Autodesk Inventor part; units mm, degrees
ref_plane "YZ Plane" through (0, 0, 0) normal (1, 0, 0) x (0, 1, 0)
ref_plane "XZ Plane" through (0, 0, 0) normal (0, 1, 0) x (-1, 0, 0)
ref_plane "XY Plane" through (0, 0, 0) normal (0, 0, 1) x (1, 0, 0)
sketch "Sketch1" plane through (0, 0, 0) normal (0, 0, 1) x (1, 0, 0)
  line L0 (55, -30) -> (-55, -30)
  line L1 (-55, -30) -> (-55, 30)
  line L2 (-55, 30) -> (55, 30)
  line L3 (55, 30) -> (55, -30)
  line L4 (49.5, -24.5) -> (-49.5, -24.5)
  line L5 (-49.5, -24.5) -> (-49.5, 24.5)
  line L6 (-49.5, 24.5) -> (49.5, 24.5)
  line L7 (49.5, 24.5) -> (49.5, -24.5)
  line L8 (55, 0) -> (-55, 0) construction
  line L9 (0, -30) -> (0, 30) construction
  line L10 (-35, 30) -> (-35, 24.5)
  line L11 (-55, 15) -> (-49.5, 15)
  line L12 (35, -24.5) -> (35, -30)
  line L13 (49.5, -15) -> (55, -15)
  line L14 (-35, -24.5) -> (-35, -30)
  line L15 (-55, -15) -> (-49.5, -15)
  line L16 (35, 30) -> (35, 24.5)
  line L17 (49.5, 15) -> (55, 15)
  line L18 (-52.25, 27.25) -> (52.25, 27.25) construction
  line L19 (52.25, 27.25) -> (52.25, -27.25) construction
  line L20 (52.25, -27.25) -> (-52.25, -27.25) construction
  line L21 (-52.25, -27.25) -> (-52.25, 27.25) construction
  line L22 (-52.25, 27.25) -> (52.25, -27.25) construction
  line L23 (52.25, 27.25) -> (-52.25, -27.25) construction
  point P0 (0, 0)
  point P1 (-35.5, 20)
  point P2 (35.5, 20)
  point P3 (35.5, -20)
  point P4 (-35.5, -20)
  dimension "d0" = 110
  dimension "d1" = 60
  dimension "d2" = 99
  dimension "d3" = 49
  dimension "d4" = 15
  dimension "d5" = 20
  dimension "d6" = 40
  dimension "d7" = 71
extrude "Extrusion1" add sketch "Sketch1" against normal blind 40 contours L0 L12 L4 L7 L13 L3 | L0 L1 L15 L5 L4 L14 | L17 L7 L6 L16 L2 L3 | L1 L2 L10 L6 L5 L11
extrude "Extrusion2" add sketch "Sketch1" along normal blind 10
hole "Hole1" at (-35.5, 20, 0) at (35.5, 20, 0) at (35.5, -20, 0) at (-35.5, -20, 0) direction (0, 0, 1) diameter 3.2 end through all counterbore diameter 6 counterbore depth 5
extrude "Extrusion8" add sketch "Sketch1" against normal blind 20 contours L0 L14 L4 L12 | L13 L7 L17 L3 | L1 L11 L5 L15 | L16 L6 L10 L2
equation "\"epsilon\" = 0"
properties part number "magnet_holder" material "PC/ABS Plastic"
Work out the finished part from the listing and answer in its coordinate system (mm). A direction names the side the tool comes from. Round coordinates to 2 decimals unless told otherwise and drop trailing zeros. Loops run counter-clockwise (first coordinate to the right, second up) from the corner with the lowest first, then second, coordinate; pieces in that order, holes last.
(1) The mould has two halves that part along X. Classify faces 4 (the flat face through (52, 0, -20)), 5 (the flat face through (55, 0, -9)), 6 (the flat face through (-34, 21, 5)): pulls with the +X half, pulls with the -X half, needs draft (parallel to the pull), parting line crosses it, or undercut.
Computed values:
face 4: needs draft
face 5: pulls with the +X half
face 6: undercut
(2) Find the intervals of material crossed by L1, parallel to X at y = 20, z = 8; L2, parallel to X at y = -20, z = 2.6; L3, parallel to Y at x = 7, z = -15, in increasing order.
Computed values:
L1: x = -55 to -37.1, -33.9 to 33.9, 37.1 to 55
L2: x = -55 to -38.5, -32.5 to 32.5, 38.5 to 55
L3: y = -30 to -24.5, 24.5 to 30
(3) The part is cut by section C-C, the plane x = 25.5. Give the vertices of the cut face in (y, z), and give its area (3 significant figures).
Computed values:
outline: (-30, -20) - (-24.5, -20) - (-24.5, 0) - (24.5, 0) - (24.5, -20) - (30, -20) - (30, 10) - (-30, 10) - close
area: 820 mm2
(4) The part is cut by section A-A, the plane y = 20. Give the vertices of the cut face in (x, z).
Computed values:
outline: (-55, -40) - (-49.5, -40) - (-49.5, 0) - (-38.5, 0) - (-38.5, 5) - (-37.1, 5) - (-37.1, 10) - (-55, 10) - close; (-33.9, 5) - (-32.5, 5) - (-32.5, 0) - (32.5, 0) - (32.5, 5) - (33.9, 5) - (33.9, 10) - (-33.9, 10) - close; (37.1, 5) - (38.5, 5) - (38.5, 0) - (49.5, 0) - (49.5, -40) - (55, -40) - (55, 10) - (37.1, 10) - close
(5) The part is cut by section B-B, the plane z = -13.5. Give the vertices of the cut face in (x, y), and give its area (3 significant figures).
Computed values:
outline: (-55, -30) - (55, -30) - (55, 30) - (-55, 30) - close; hole (-49.5, -24.5) - (49.5, -24.5) - (49.5, 24.5) - (-49.5, 24.5) - close
area: 1,750 mm2
(6) For faces 1 (the cylindrical face through (33.47, -22.21, 2.54)), 2 (the flat face through (52, -15, -30)), 3 (the cylindrical face through (37.06, -20.35, 7.54)), determine the directions among +Z, -Z, +X, -X, +Y, -Y from which every point of the face is accessible in a straight line to the end or side of a thin tool.
Computed values:
face 1: -Z
face 2: -Z, +X, -X
face 3: +Z, -Z
(7) Each of these flat-tipped pins is pushed along its axis until it touches: P1, Ø3, axis at x = -51.5, y = -3.5, coming from the -Z side; P2, Ø1.8, axis at x = -34, y = 20, coming from the -Z side; P3, Ø1, axis at x = 17.5, y = -7.5, coming from the -Z side; P4, Ø12, axis at y = -8, z = -22.5, coming from the +X side. Where does it stop, or does it pass through?
Computed values:
P1: stops at z = -20
P2: stops at z = 5
P3: stops at z = 0
P4: stops at x = 55
(8) The part is cut by section D-D, the plane y = 0. Give the vertices of the cut face in (x, z).
Computed values:
outline: (-55, -20) - (-49.5, -20) - (-49.5, 0) - (49.5, 0) - (49.5, -20) - (55, -20) - (55, 10) - (-55, 10) - close
